Can you work these out from the model? Positions are in its coordinate system, mm. Face numbers are marked on the shaded views. A direction names the side the tool comes from. Coordinates: 2 decimals unless noted, no trailing zeros. Write each loop counter-clockwise with the first axis right and the second up, starting at its lowest first coordinate (ties: lowest second). Pieces come first, ordered by that corner, then holes. Notation, with made-up numbers: (9, 47) - (14, 47) arc R29 cw to (14, 78) - close; hole circle Ø8 at (-30, 83). An arc over 180 degrees is marked (long way). One line per question, with ' | ' between items. Start each with the question number.
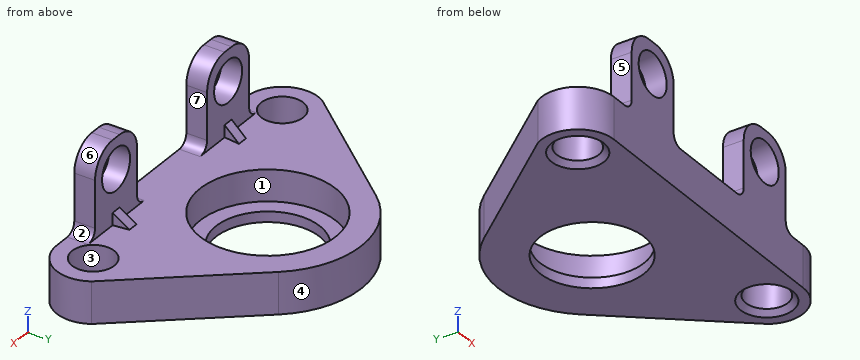
from build123d import *

# Parameters (mm, degrees)
SALIENTE_EXTRUIR1_DEPTH = 23
SALIENTE_EXTRUIR2_DEPTH = 2
CROQUIS3_W              = 74.8935
CROQUIS3_H              = 50
SALIENTE_EXTRUIR3_DEPTH = 2
CROQUIS4_R              = 4.05
SALIENTE_EXTRUIR4_DEPTH = 50
CHAFL_N2_SIZE           = 1
CROQUIS7_R              = 4.05
CROQUIS7_R_2            = 13.05
SALIENTE_EXTRUIR5_DEPTH = 6
CROQUIS8_W              = 12
CROQUIS8_H              = 4
SALIENTE_EXTRUIR6_DEPTH = 16
REDONDEO3_R             = 2
REDONDEO4_R             = 5
CROQUIS14_R             = 4
CORTAR_EXTRUIR1_DEPTH   = 10
SALIENTE_EXTRUIR7_DEPTH = 1
CROQUIS20_R             = 4.05
CROQUIS20_R_2           = 10
SALIENTE_EXTRUIR8_DEPTH = 2
CHAFL_N3_SIZE           = 1


with BuildPart() as part:
    # Croquis1 → Saliente-Extruir1 (new, symmetric)
    with BuildSketch(Plane.XY):
        Polygon((-7.48935, 0), (7.48935, 0), (0.00065, 21.6199), align=None)
    extrude(amount=SALIENTE_EXTRUIR1_DEPTH, both=True)

    # Croquis2 → Saliente-Extruir2 (add)
    with BuildSketch(Plane.XY.offset(23)):
        Polygon((37.44675, 0), (-37.44675, 0), (0.00065, 21.6199), align=None)
    saliente_extruir2 = extrude(amount=SALIENTE_EXTRUIR2_DEPTH)

    # Simetría1: Saliente-Extruir2 across plane
    add(saliente_extruir2.mirror(Plane.XY))

    # Croquis3 → Saliente-Extruir3 (add)
    with BuildSketch(Plane.XZ):
        Rectangle(CROQUIS3_W, CROQUIS3_H)
    extrude(amount=SALIENTE_EXTRUIR3_DEPTH)

    # Croquis4 → Saliente-Extruir4 (add)
    with BuildSketch(Plane.XY.offset(25)):
        with BuildLine():
            Line((7.743545699, -2), (-7.743545699, -2))
            ThreePointArc((-7.743545699, -2), (-6.147743753, -2.794422898), (-5.819683414, -4.546583851))
            ThreePointArc((-5.819683414, -4.546583851), (0, -12.25), (5.819683414, -4.546583851))
            ThreePointArc((5.819683414, -4.546583851), (6.147743753, -2.794422898), (7.743545699, -2))
        make_face()
        with Locations((0, -6.2)):
            Circle(CROQUIS4_R, mode=Mode.SUBTRACT)
    extrude(amount=-SALIENTE_EXTRUIR4_DEPTH)

    # Chaflán2
    chafl_n2_edges = [part.edges().sort_by_distance(p)[0] for p in [
        (-4.05, -6.2, -25),
        (-4.05, -6.2, 25),
    ]]
    chamfer(chafl_n2_edges, length=CHAFL_N2_SIZE)


with BuildPart() as body_2:
    # Croquis7 → Saliente-Extruir5 (new body)
    with BuildSketch(Plane(origin=(0, 0, -25), x_dir=(-1, 0, 0), z_dir=(0, 0, -1))):
        with BuildLine():
            Line((27, -28.615252187), (-27, -28.615252187))
            ThreePointArc((-27, -28.615252187), (-33.112686004, -25.026274001), (-32.957287229, -17.939557849))
            Line((-32.957287229, -17.939557849), (-13.903204494, 5.232449641))
            ThreePointArc((-13.903204494, 5.232449641), (0, 11.8), (13.903204494, 5.232449641))
            Line((13.903204494, 5.232449641), (32.957287229, -17.939557849))
            ThreePointArc((32.957287229, -17.939557849), (33.112686004, -25.026274001), (27, -28.615252187))
        make_face()
        with Locations((-27, -21.615252187)):
            Circle(CROQUIS7_R, mode=Mode.SUBTRACT)
        with Locations(Location((27, -21.615252187, 0), (0, 0, 180))):
            Circle(CROQUIS7_R, mode=Mode.SUBTRACT)
        with Locations((0, -6.2)):
            Circle(CROQUIS7_R_2, mode=Mode.SUBTRACT)
    extrude(amount=SALIENTE_EXTRUIR5_DEPTH)

    # Croquis8 → Saliente-Extruir6 (add)
    with BuildSketch(Plane.XY.offset(-25)):
        with Locations((-16, -26.615252187)):
            Rectangle(CROQUIS8_W, CROQUIS8_H)
        with Locations((16, -26.615252187)):
            Rectangle(CROQUIS8_W, CROQUIS8_H)
    extrude(amount=SALIENTE_EXTRUIR6_DEPTH)

    # Redondeo3
    redondeo3_edges = [body_2.edges().sort_by_distance(p)[0] for p in [
        (-22, -26.615252187, -25),
        (-10, -26.615252187, -25),
        (22, -26.615252187, -25),
        (10, -26.615252187, -25),
    ]]
    fillet(redondeo3_edges, radius=REDONDEO3_R)

    # Redondeo4
    redondeo4_edges = [body_2.edges().sort_by_distance(p)[0] for p in [
        (-22, -26.615252187, -9),
        (-10, -26.615252187, -9),
        (22, -26.615252187, -9),
        (10, -26.615252187, -9),
    ]]
    fillet(redondeo4_edges, radius=REDONDEO4_R)

    # Croquis14 → Cortar-Extruir1 (cut)
    with BuildSketch(Plane(origin=(0, -24.615252187, 0), x_dir=(1, 0, 0), z_dir=(0, 1, 0))):
        with Locations(Location((-16, 15, 0), (0, 0, 270))):
            Circle(CROQUIS14_R)
        with Locations(Location((16, 15, 0), (0, 0, 270))):
            Circle(CROQUIS14_R)
    extrude(amount=-CORTAR_EXTRUIR1_DEPTH, mode=Mode.SUBTRACT)

    # Croquis3D2 → Saliente-Extruir7 (add, symmetric, along a direction that is not the sketch's normal)
    with BuildSketch(Plane(origin=(-16, -24.615252187, -22.681195735), x_dir=(0.09307928640942055, 0.7877707078361105, -0.6088953590863595), z_dir=(-0.9930919098636288, 0.11733907517707019, 0))):
        Polygon((0, 0), (3.808214713, 0), (1.411909156, 1.839392768), align=None)
    saliente_extruir7 = extrude(amount=SALIENTE_EXTRUIR7_DEPTH, dir=(-1, 0, 0), both=True)

    # Simetría2: Saliente-Extruir7 across plane
    add(saliente_extruir7.mirror(Plane(origin=(0, 0, 0), x_dir=(0, 0, 1), z_dir=(1, 0, 0))))

    # Croquis20 → Saliente-Extruir8 (add)
    with BuildSketch(Plane(origin=(0, 0, -31), x_dir=(-1, 0, 0), z_dir=(0, 0, -1))):
        with BuildLine():
            Line((32.957287229, -17.939557849), (13.903204494, 5.232449641))
            ThreePointArc((13.903204494, 5.232449641), (0, 11.8), (-13.903204494, 5.232449641))
            Line((-13.903204494, 5.232449641), (-32.957287229, -17.939557849))
            ThreePointArc((-32.957287229, -17.939557849), (-33.112686004, -25.026274001), (-27, -28.615252187))
            Line((-27, -28.615252187), (27, -28.615252187))
            ThreePointArc((27, -28.615252187), (33.112686004, -25.026274001), (32.957287229, -17.939557849))
        make_face()
        with Locations((-27, -21.615252187)):
            Circle(CROQUIS20_R, mode=Mode.SUBTRACT)
        with Locations(Location((27, -21.615252187, 0), (0, 0, 180))):
            Circle(CROQUIS20_R, mode=Mode.SUBTRACT)
        with Locations((0, -6.2)):
            Circle(CROQUIS20_R_2, mode=Mode.SUBTRACT)
    extrude(amount=SALIENTE_EXTRUIR8_DEPTH)

    # Chaflán3
    chafl_n3_edges = [body_2.edges().sort_by_distance(p)[0] for p in [
        (31.05, -21.615252187, -33),
        (-31.05, -21.615252187, -33),
    ]]
    chamfer(chafl_n3_edges, length=CHAFL_N3_SIZE)


solid = body_2.part
(1) If we section it at A-A on z = -15: List the corners of the cut face in (x, y) for me.
(2) I'm going to push flat-ended pins straight in: pin 1 (10 mm diameter, centred on y = -8.5, z = -26.5, fed in from -X); pin 2 (10 mm diameter, centred on y = -2.5, z = -26, fed in from -X); pin 3 (1 mm diameter, centred on x = 21, z = -16, fed in from +Y). Where does each tip first touch, or does it pass through?
(3) If we section it at D-D on y = -13: List the corners of the cut face in (x, z) for me.
(4) If we mould it in two halves opening along Y, with no side actions, what happens to the marked faces 1, 2, 3 and 4? For each: +Y half, -Y half, draft (parallel to the pull), parting line (faces both ways), or undercut.
(5) If we section it at B-B on z = -27.75: List the corners of the cut face in (x, y) for me.
(6) Which directions (+Z, -Z, +X, -X, +Y, -Y) give clear straight access to the entire face, cutting with the end or side of a thin tool? Please do the marked faces 5, 6 and 7.
(7) If we section it at C-C on x = 2: List the corners of the cut face in (y, z) for me.
(8) If I drill on probe 1 along X at (y, z) = (-25.45, -15); probe 2 along Y at (x, z) = (0, -27.55); probe 3 along Y at (x, z) = (-19.5, -23.5), over which ranges is the centre line in solid material (lowest first)?
Values:
1) outline: (-22, -28.62) - (-20, -28.62) - (-20, -24.62) - (-22, -24.62) - close; (-12, -28.62) - (-10, -28.62) - (-10, -24.62) - (-12, -24.62) - close; (10, -28.62) - (12, -28.62) - (12, -24.62) - (10, -24.62) - close; (20, -28.62) - (22, -28.62) - (22, -24.62) - (20, -24.62) - close
2) pin 1: x = -29.31 | pin 2: x = -24.37 | pin 3: y = -24.62
3) outline: (-28.9, -33) - (-7.33, -33) - (-7.33, -31) - (-11.14, -31) - (-11.14, -25) - (-28.9, -25) - close; (7.33, -33) - (28.9, -33) - (28.9, -25) - (11.14, -25) - (11.14, -31) - (7.33, -31) - close
4) face 1: undercut | face 2: draft | face 3: undercut | face 4: +Y half
5) outline: (-32.96, -17.94) arc R7 ccw to (-27, -28.62) - (27, -28.62) arc R7 ccw to (32.96, -17.94) - (13.9, 5.23) arc R18 ccw to (-13.9, 5.23) - close; hole circle Ø8.1 at (-27, -21.62); hole circle Ø26.1 at (0, -6.2); hole circle Ø8.1 at (27, -21.62)
6) face 5: +Z, -X, +Y, -Y | face 6: +Z, +X, +Y, -Y | face 7: +Z, +Y, -Y
7) outline: (-28.62, -33) - (-16, -33) - (-16, -31) - (-19.1, -31) - (-19.1, -25) - (-28.62, -25) - close; (3.6, -33) - (11.69, -33) - (11.69, -25) - (6.7, -25) - (6.7, -31) - (3.6, -31) - close
8) probe 1: -22 to -20, -12 to -10, 10 to 12, 20 to 22 | probe 2: -28.62 to -19.25, 6.85 to 11.8 | probe 3: -28.62 to -24.62
